```python
from build123d import *

# Parameters (mm, degrees)
SKETCH1_W           = 76.2
SKETCH1_H           = 152.4
SKETCH1_R           = 2.7305
SKETCH1_R_2         = 1.8288
BOSS_EXTRUDE1_DEPTH = 6.35


with BuildPart() as part:
    # Sketch1 → Boss-Extrude1 (new body)
    with BuildSketch(Plane(origin=(0, 0, 0), x_dir=(1, 0, 0), z_dir=(0, 1, 0))):
        Rectangle(SKETCH1_W, SKETCH1_H)
        with Locations((0, 57.15)):
            Circle(SKETCH1_R, mode=Mode.SUBTRACT)
        with Locations((0, 19.05)):
            Circle(SKETCH1_R, mode=Mode.SUBTRACT)
        with Locations((0, -19.05)):
            Circle(SKETCH1_R, mode=Mode.SUBTRACT)
        with Locations((0, -57.15)):
            Circle(SKETCH1_R, mode=Mode.SUBTRACT)
        with Locations((27.305, 38.1)):
            Circle(SKETCH1_R_2, mode=Mode.SUBTRACT)
        with Locations((27.305, 0)):
            Circle(SKETCH1_R_2, mode=Mode.SUBTRACT)
        with Locations((27.305, -38.1)):
            Circle(SKETCH1_R_2, mode=Mode.SUBTRACT)
        with Locations((-27.305, 0)):
            Circle(SKETCH1_R_2, mode=Mode.SUBTRACT)
        with Locations((-27.305, -38.1)):
            Circle(SKETCH1_R_2, mode=Mode.SUBTRACT)
        with Locations((-27.305, 38.1)):
            Circle(SKETCH1_R_2, mode=Mode.SUBTRACT)
    extrude(amount=-BOSS_EXTRUDE1_DEPTH)


solid = part.part
```
Model file for the job. Use its own axes, mm. Coordinates: 2 decimals unless noted, no trailing zeros. Loops run counter-clockwise (first coordinate to the right, second up) from the corner with the lowest first, then second, coordinate; pieces in that order, holes last. Notation, with made-up numbers: (87, 43) - (117, 43) arc R21 cw to (117, 67) - close; hole circle Ø11 at (76.25, 6). An arc over 180 degrees is marked (long way). Answer as a JSON object with one key per item and string values. Group by question number.
(1) Cut at A-A (z = -19.05). Give the cut face in (x, y).
(2) Probe line 1 along Z through (x, y) = (0, -0.25); line 2 along X through (y, z) = (-3.5, 0); line 3 along Z through (x, y) = (27.5, -3). List the from-to ranges inside material, lowest first.
(3) Cut at C-C (z = 38.1). Give the cut face in (x, y), then the cut area to 3 significant figures.
(4) Two-plate mould, pull along Z, no slides. Class faces 1 (the face through (-0.592, -3.131, -54.484)), 2 (the face through (-1, -3, -76.2)), 3 (the face through (-1, 0, -1)), 4 (the face through (-1, -3, 76.2)): released by +Z, released by -Z, zero draft, split by the parting line, or undercut.
(5) Cut at B-B (x = 0). Give the cut face in (y, z), then the cut area to 3 significant figures.
(6) Flat gauge pin, fed straight in: pin 1 (5 mm diameter, centred on x = 0, z = -19.05, fed in from +Y). Where does the tip first touch, or does it go through?
Geometry says:
{
 "1": {"outline": "(-38.1, -6.35) - (-2.73, -6.35) - (-2.73, 0) - (-38.1, 0) - close; (2.73, -6.35) - (38.1, -6.35) - (38.1, 0) - (2.73, 0) - close"},
 "2": {"line 1": "z = -76.2 to -59.88, -54.42 to -21.78, -16.32 to 16.32, 21.78 to 54.42, 59.88 to 76.2", "line 2": "x = -38.1 to -29.13, -25.48 to 25.48, 29.13 to 38.1", "line 3": "z = -76.2 to -39.92, -36.28 to -1.82, 1.82 to 36.28, 39.92 to 76.2"},
 "3": {"outline": "(-38.1, -6.35) - (-29.13, -6.35) - (-29.13, 0) - (-38.1, 0) - close; (-25.48, -6.35) - (25.48, -6.35) - (25.48, 0) - (-25.48, 0) - close; (29.13, -6.35) - (38.1, -6.35) - (38.1, 0) - (29.13, 0) - close", "area": "437 mm^2"},
 "4": {"face 1": "undercut", "face 2": "released by -Z", "face 3": "zero draft", "face 4": "released by +Z"},
 "5": {"outline": "(-6.35, -76.2) - (0, -76.2) - (0, -59.88) - (-6.35, -59.88) - close; (-6.35, -54.42) - (0, -54.42) - (0, -21.78) - (-6.35, -21.78) - close; (-6.35, -16.32) - (0, -16.32) - (0, 16.32) - (-6.35, 16.32) - close; (-6.35, 21.78) - (0, 21.78) - (0, 54.42) - (-6.35, 54.42) - close; (-6.35, 59.88) - (0, 59.88) - (0, 76.2) - (-6.35, 76.2) - close", "area": "829 mm^2"},
 "6": {"pin 1": "passes through"}
}
